from build123d import *

# Parameters (mm, degrees)
SKETCH_1_R          = 23.14
EXTRUDE_1_DEPTH     = 1.25
SKETCH_2_R          = 20.2
EXTRUDE_2_DEPTH     = 1.75
CUT_EXTRUDE_1_DEPTH = 1.75
CUT_EXTRUDE_START   = 1.25
SKETCH_5_R          = 1.20000014
SKETCH_5_R_2        = 5.3
CUT_EXTRUDE_2_DEPTH = 3
CHAMFER_1_SIZE      = 3.5
CHAMFER_1_SIZE2     = 0.8
CHAMFER_2_SIZE      = 0.5
CUT_EXTRUDE_START_2 = -1.75
CUT_EXTRUDE_3_DEPTH = 1.3


with BuildPart() as part:
    # 草图1 → 凸台-拉伸1 (new body)
    with BuildSketch(Plane.XY):
        with Locations((91.99900066, 78.41000066)):
            Circle(SKETCH_1_R)
    extrude(amount=EXTRUDE_1_DEPTH)

    # 草图2 → 凸台-拉伸2 (add)
    with BuildSketch(Plane.XY):
        with Locations((91.99900066, 78.41000066)):
            Circle(SKETCH_2_R)
    extrude(amount=-EXTRUDE_2_DEPTH)

    # 草图3 → 切除-拉伸1 (cut)
    with BuildSketch(Plane.XY):
        with BuildLine():
            Line((99.695, 96.266), (99.695, 97.658416258))
            ThreePointArc((99.695, 97.658416258), (92.012378583, 99.139588259), (84.327969421, 97.66771932))
            Line((84.327969421, 97.66771932), (84.327969421, 94.233969421))
            Line((84.327969421, 94.233969421), (84.074, 93.98))
            Line((84.074, 93.98), (79.629, 93.98))
            Line((79.629, 93.98), (79.248, 93.599))
            Line((79.248, 93.599), (79.248, 91.059))
            Line((79.248, 91.059), (78.74, 90.551))
            Line((78.74, 90.551), (78.74, 88.138))
            Line((78.74, 88.138), (79.121, 87.757))
            Line((79.121, 87.757), (83.566, 87.757))
            Line((83.566, 87.757), (84.201, 87.122))
            Line((84.201, 87.122), (84.201, 85.471))
            Line((84.201, 85.471), (84.455, 85.217))
            Line((84.455, 85.217), (86.233, 85.217))
            Line((86.233, 85.217), (86.752296117, 84.697830406))
            Line((86.752296117, 84.697830406), (96.762680157, 84.697680157))
            Line((96.762680157, 84.697680157), (97.282, 85.217))
            Line((97.282, 85.217), (99.314, 85.217))
            Line((99.314, 85.217), (99.568, 85.471))
            Line((99.568, 85.471), (99.568, 85.725))
            Line((99.568, 85.725), (99.568, 86.741))
            Line((99.568, 86.741), (99.695, 86.868))
            Line((99.695, 86.868), (104.14, 86.868))
            Line((104.14, 86.868), (104.648, 87.376))
            Line((104.648, 87.376), (104.648, 93.472))
            Line((104.648, 93.472), (104.14, 93.98))
            Line((104.14, 93.98), (101.854, 93.98))
            Line((101.854, 93.98), (101.6, 94.234))
            Line((101.6, 94.234), (101.6, 95.631))
            Line((101.6, 95.631), (101.219, 96.012))
            Line((101.219, 96.012), (99.949, 96.012))
            Line((99.949, 96.012), (99.695, 96.266))
        make_face()
    extrude(amount=-CUT_EXTRUDE_1_DEPTH, mode=Mode.SUBTRACT)

    # 草图5 → 切除-拉伸2 (cut)
    with BuildSketch(Plane.XY.offset(CUT_EXTRUDE_START)):
        with Locations((104.267, 78.41000066)):
            Circle(SKETCH_5_R)
        with Locations((91.99900066, 78.41000066)):
            Circle(SKETCH_5_R_2)
    extrude(amount=-CUT_EXTRUDE_2_DEPTH, mode=Mode.SUBTRACT)

    # 倒角1
    chamfer_1_edges = [part.edges().sort_by_distance(p)[0] for p in [
        (103.06699986, 78.41000066, 1.25),
    ]]
    chamfer_1_side = [part.faces().sort_by_distance(p)[0] for p in [
        (69.513498697, 78.41000066, 1.25),
    ]]
    chamfer(chamfer_1_edges, length=CHAMFER_1_SIZE, length2=CHAMFER_1_SIZE2, reference=chamfer_1_side[0])

    # 倒角2
    chamfer_2_edges = [part.edges().sort_by_distance(p)[0] for p in [
        (86.69900066, 78.41000066, 1.25),
    ]]
    chamfer(chamfer_2_edges, length=CHAMFER_2_SIZE)

    # 草图6 → 切除-拉伸3 (cut)
    with BuildSketch(Plane.XY.offset(CUT_EXTRUDE_START_2)):
        Polygon((101.727, 82.931), (101.346, 82.55), (101.346, 74.422), (101.6, 74.168), (106.68, 74.168), (107.315, 74.803), (107.315, 82.423), (106.807, 82.931), align=None)
    extrude(amount=CUT_EXTRUDE_3_DEPTH, mode=Mode.SUBTRACT)


solid = part.part
Geometry check sheet. Reference: the model listing, model coordinates, mm. A direction names the side the tool comes from. Give positions to 0.01 mm unless a question says otherwise; leave off trailing zeros. Write each loop counter-clockwise with the first axis right and the second up, starting at its lowest first coordinate (ties: lowest second). Pieces come first, ordered by that corner, then holes.
1) Cross-section at B-B (x = 74). Record the boundary of the cut face in (y, z).
Values follow:
outline: (63.87, 0) - (69.24, 0) - (69.24, -1.75) - (87.58, -1.75) - (87.58, 0) - (92.95, 0) - (92.95, 1.25) - (63.87, 1.25) - close
2) Set-up check for faces 4 (the face through (97, 74, 1.25)), 5 (the face through (99.568, 86, -1)), 6 (the face through (101.346, 79, -1)): record each of +Z, -Z, +X, -X, +Y, -Y from which the full face is reachable in a straight line by a thin tool's end or side.
Values follow:
face 4: +Z, +X, -X, +Y, -Y
face 5: -Z, +Y
face 6: -Z
3) Go/stop test with flat-tipped pins: pin 1 Ø0.5 at (y, z) = (89, -0.5) entering from +X; pin 2 Ø0.9 at (y, z) = (92.5, -1) entering from +X; pin 3 Ø1.5 at (x, z) = (89, -0.5) entering from +Y. Record where each tip stops, or that it passes through.
Values follow:
pin 1: stops at x = 109.35
pin 2: stops at x = 106.9
pin 3: stops at y = 101.42
4) Release check for a two-part mould opening along Y. For faces 1 (the face through (86.98, 55.82, 0.62)), 2 (the face through (107.315, 79, -1)), 3 (the face through (84.328, 96, -1)) record: released by +Y, released by -Y, zero draft, split by the parting line, or undercut.
Values follow:
face 1: split by the parting line
face 2: undercut
face 3: zero draft
5) Cross-section at A-A (y = 78.41). Count the separate pieces of the cut face and the enclosed holes in it, plus the area to 3 significant figures.
Values follow:
separate pieces: 3
enclosed holes: 0
area: 81.9 mm2
6) Thickness scan on line 1 (X direction, y = 81, z = 0.6); line 2 (Y direction, x = 104, z = -0.1); line 3 (Z direction, x = 77, y = 93). Record the ranges inside material, lowest first.
Values follow:
line 1: x = 69 to 87.37, 96.62 to 114.99
line 2: y = 62.16 to 77.24, 79.58 to 86.87, 93.98 to 94.66
line 3: z = 0 to 1.25
7) Cross-section at C-C (y = 71). Record the boundary of the cut face in (x, z).
Values follow:
outline: (70.08, 0) - (73.21, 0) - (73.21, -1.75) - (110.79, -1.75) - (110.79, 0) - (113.92, 0) - (113.92, 1.25) - (70.08, 1.25) - close
